Here's the drawing with two shaded views (mm, measured from the low corner). I have some questions. Give positions to 0.01 mm unless a question says otherwise; leave off trailing zeros. Write each loop counter-clockwise with the first axis right and the second up, starting at its lowest first coordinate (ties: lowest second). Pieces come first, ordered by that corner, then holes. Notation, with made-up numbers: M 67.25,-38.5 L 120.25,-38.5 A9 cw 120.25,-27.5 Z; hole C -17,83.25 d3. An arc over 180 degrees is marked long. Answer as a JSON object with one key per item and string values. Group by question number.
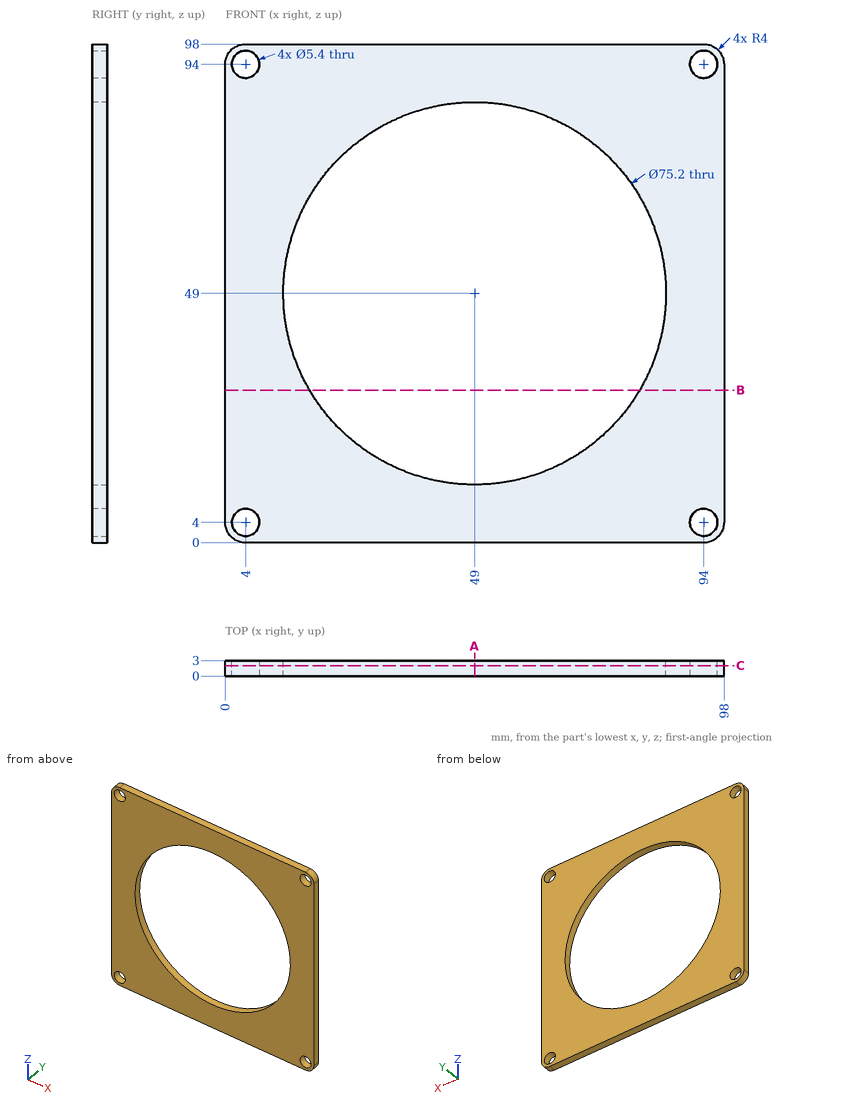
1) If we section it at A-A, the plane x = 49: List the corners of the cut face in (y, z) for me, plus the area to 3 significant figures.
2) Please list where these lines run through material, in increasing order: line 1 along Z through (x, y) = (94, 2.2); line 2 along X through (y, z) = (1.55, 50). Write a range as from..to.
3) If we section it at B-B, the plane z = 30: List the corners of the cut face in (x, y) for me, plus the area to 3 significant figures.
4) If we section it at C-C, the plane y = 2.05: List the corners of the cut face in (x, z) for me, plus the area to 3 significant figures.
Taken from the geometry:
{
 "1": {"outline": "M 0,0 L 3,0 L 3,11.4 L 0,11.4 Z; M 0,86.6 L 3,86.6 L 3,98 L 0,98 Z", "area": "68.4 mm²"},
 "2": {"line 1": "0..1.3, 6.7..91.3, 96.7..98", "line 2": "0..11.41, 86.59..98"},
 "3": {"outline": "M 0,0 L 16.55,0 L 16.55,3 L 0,3 Z; M 81.45,0 L 98,0 L 98,3 L 81.45,3 Z", "area": "99.3 mm²"},
 "4": {"outline": "M 0,4 A4 ccw 4,0 L 94,0 A4 ccw 98,4 L 98,94 A4 ccw 94,98 L 4,98 A4 ccw 0,94 Z; hole C 4,4 d5.4; hole C 4,94 d5.4; hole C 49,49 d75.2; hole C 94,4 d5.4; hole C 94,94 d5.4", "area": "5,060 mm²"}
}
